Part print with two shaded views. Sizes in mm from the minimum x, y, z corner. A direction names the side the tool comes from. Give positions to 0.01 mm unless a question says otherwise; leave off trailing zeros. Order: outer loops, then holes, each group sorted by start corner. A loop starts at its lowest first (then second) coordinate and runs counter-clockwise, first axis right, second up. Notation, with made-up numbers: M 88,78.25 L 132,78.25 A11 ccw 132,95.25 Z; hole C -37.75,69 d10. An arc over 180 degrees is marked long. Return JSON: item names as keys, results as strings. Group by question number.
1. 3-axis set-ups, long thin cutter, end or side, ignore diameter. For the marked faces 1, 2, 3 and 4: which of +Z, -Z, +X, -X, +Y, -Y reach the whole face in a straight line?
2. Slice it at B-B on y = 109.5. List the corners of the cut face in (x, z) (1 decimal).
3. Slice it at D-D on x = 41. List the corners of the cut face in (y, z) (1 decimal).
4. Wall check: probe 1 along Y at (x, z) = (52.5, 33) (1 decimal); probe 2 along Z at (x, y) = (28, 50); probe 3 along X at (y, z) = (117, 55.5) (1 decimal). Give the ranges that are in metal, low to high. Write a range as [from, to].
5. Pin check, flat tips, straight feed: pin 1 (2 mm diameter, centred on x = 35.5, y = 56.5, fed in from +Z); pin 2 (3.5 mm diameter, centred on x = 71, z = 9, fed in from +Y); pin 3 (22 mm diameter, centred on x = 19, z = 55.5, fed in from -Y). Stop position of each tip, or through.
6. Slice it at A-A on z = 61.5. List the corners of the cut face in (x, y) (1 decimal), then the cut area to 3 significant figures.
7. Slice it at C-C on x = 64.5. List the corners of the cut face in (y, z) (1 decimal).
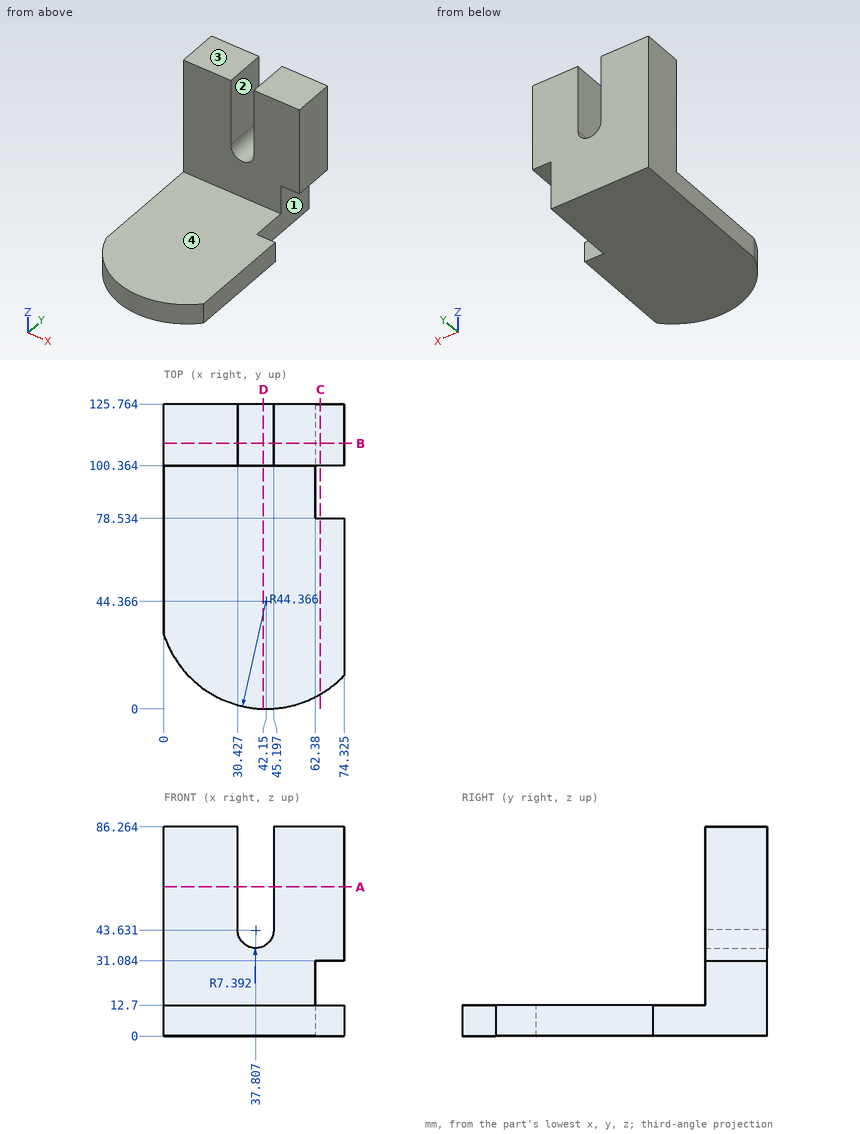
Result:
{
 "1": {"face 1": "-Z, +X, +Y", "face 2": "+Z, +Y, -Y", "face 3": "+Z, +X, -X, +Y, -Y", "face 4": "+Z, +X, -X, -Y"},
 "2": {"outline": "M 0,0 L 62.4,0 L 62.4,31.1 L 74.3,31.1 L 74.3,86.3 L 45.2,86.3 L 45.2,43.8 A7.4 cw long 30.4,44 L 30.4,86.3 L 0,86.3 Z"},
 "3": {"outline": "M 0,0 L 125.8,0 L 125.8,37 L 100.4,37 L 100.4,12.7 L 0,12.7 Z"},
 "4": {"probe 1": "y = [100.4, 125.8]", "probe 2": "z = [0, 12.7]", "probe 3": "x = [0, 30.4], [45.2, 74.3]"},
 "5": {"pin 1": "stops at z = 12.7", "pin 2": "stops at y = 78.53", "pin 3": "stops at y = 100.36"},
 "6": {"outline": "M 0,100.4 L 30.4,100.4 L 30.4,125.8 L 0,125.8 Z; M 45.2,100.4 L 74.3,100.4 L 74.3,125.8 L 45.2,125.8 Z", "area": "1,510 mm2"},
 "7": {"outline": "M 6,0 L 78.5,0 L 78.5,12.7 L 6,12.7 Z; M 100.4,31.1 L 125.8,31.1 L 125.8,86.3 L 100.4,86.3 Z"}
}
